Input: part model. Units: mm. Frame: model coordinates. Coordinates: 2 decimals unless noted, no trailing zeros. Order: outer loops, then holes, each group sorted by start corner. A loop starts at its lowest first (then second) coordinate and runs counter-clockwise, first axis right, second up. Notation, with made-up numbers: (34.25, 11.25) - (42.25, 11.25) arc R19 ccw to (42.25, 22.25) - close; hole circle Ø3 at (-21.5, 8.25). An arc over 180 degrees is marked (long way). One line per question, with ' | ' between items.
from build123d import *

# Parameters (mm, degrees)
SKETCH1_W           = 112
SKETCH1_H           = 70
SKETCH1_R           = 1.5
BOSS_EXTRUDE1_DEPTH = 6
SKETCH2_R           = 1.5
CUT_EXTRUDE1_DEPTH  = 85.504437753
SKETCH3_W           = 14
SKETCH3_H           = 6
CUT_EXTRUDE2_DEPTH  = 85.504437753
SKETCH4_R           = 1.5
CUT_EXTRUDE3_DEPTH  = 85.504437753
SKETCH5_R           = 12
CUT_EXTRUDE4_DEPTH  = 85.504437753
SKETCH6_R           = 1.5
CUT_EXTRUDE5_DEPTH  = 10
SKETCH7_W           = 40
SKETCH7_H           = 27.8
BOSS_EXTRUDE2_DEPTH = 6
SKETCH8_W           = 12
SKETCH8_H           = 6
CUT_EXTRUDE6_DEPTH  = 6
SKETCH9_R           = 1.5
CUT_EXTRUDE7_DEPTH  = 6


with BuildPart() as part:
    # Sketch1 → Boss-Extrude1 (new body)
    with BuildSketch(Plane(origin=(0, 0, 0), x_dir=(1, 0, 0), z_dir=(0, 1, 0))):
        with Locations((0, 28)):
            Rectangle(SKETCH1_W, SKETCH1_H)
        with Locations(Location((-6.2, 0, 0), (0, 0, 270))):
            Circle(SKETCH1_R, mode=Mode.SUBTRACT)
        with Locations(Location((-38.2, 0, 0), (0, 0, 270))):
            Circle(SKETCH1_R, mode=Mode.SUBTRACT)
        with Locations(Location((-6.2, 56, 0), (0, 0, 270))):
            Circle(SKETCH1_R, mode=Mode.SUBTRACT)
        with Locations(Location((-38.2, 56, 0), (0, 0, 270))):
            Circle(SKETCH1_R, mode=Mode.SUBTRACT)
        with Locations(Location((6.2, 0, 0), (0, 0, 90))):
            Circle(SKETCH1_R, mode=Mode.SUBTRACT)
        with Locations(Location((38.2, 0, 0), (0, 0, 90))):
            Circle(SKETCH1_R, mode=Mode.SUBTRACT)
        with Locations(Location((6.2, 56, 0), (0, 0, 90))):
            Circle(SKETCH1_R, mode=Mode.SUBTRACT)
        with Locations(Location((38.2, 56, 0), (0, 0, 90))):
            Circle(SKETCH1_R, mode=Mode.SUBTRACT)
    extrude(amount=BOSS_EXTRUDE1_DEPTH)

    # Sketch2 → Cut-Extrude1 (cut, through all)
    with BuildSketch(Plane(origin=(0, 6, 0), x_dir=(1, 0, 0), z_dir=(0, 1, 0))):
        with Locations(Location((-53, 48, 0), (0, 0, 270))):
            Circle(SKETCH2_R)
        with Locations(Location((-53, 8, 0), (0, 0, 270))):
            Circle(SKETCH2_R)
        with Locations(Location((53, 8, 0), (0, 0, 270))):
            Circle(SKETCH2_R)
        with Locations(Location((53, 48, 0), (0, 0, 270))):
            Circle(SKETCH2_R)
    extrude(amount=-CUT_EXTRUDE1_DEPTH, mode=Mode.SUBTRACT)

    # Sketch3 → Cut-Extrude2 (cut, through all)
    with BuildSketch(Plane(origin=(0, 6, 0), x_dir=(1, 0, 0), z_dir=(0, 1, 0))):
        with Locations((20.2, 56)):
            Rectangle(SKETCH3_W, SKETCH3_H)
        with Locations((20.2, 0)):
            Rectangle(SKETCH3_W, SKETCH3_H)
        with Locations((-20.2, 0)):
            Rectangle(SKETCH3_W, SKETCH3_H)
        with Locations((-20.2, 56)):
            Rectangle(SKETCH3_W, SKETCH3_H)
    extrude(amount=-CUT_EXTRUDE2_DEPTH, mode=Mode.SUBTRACT)

    # Sketch4 → Cut-Extrude3 (cut, through all)
    with BuildSketch(Plane(origin=(0, 6, 0), x_dir=(1, 0, 0), z_dir=(0, 1, 0))):
        with Locations(Location((19, 9, 0), (0, 0, 270))):
            Circle(SKETCH4_R)
        with Locations(Location((19, 47, 0), (0, 0, 90))):
            Circle(SKETCH4_R)
        with Locations(Location((-19, 47, 0), (0, 0, 270))):
            Circle(SKETCH4_R)
        with Locations(Location((-19, 9, 0), (0, 0, 90))):
            Circle(SKETCH4_R)
    extrude(amount=-CUT_EXTRUDE3_DEPTH, mode=Mode.SUBTRACT)

    # Sketch5 → Cut-Extrude4 (cut, through all)
    with BuildSketch(Plane(origin=(0, 6, 0), x_dir=(1, 0, 0), z_dir=(0, 1, 0))):
        with Locations(Location((-23, 28, 0), (0, 0, 270))):
            Circle(SKETCH5_R)
        with Locations(Location((23, 28, 0), (0, 0, 270))):
            Circle(SKETCH5_R)
    extrude(amount=-CUT_EXTRUDE4_DEPTH, mode=Mode.SUBTRACT)

    # Sketch6 → Cut-Extrude5 (cut)
    with BuildSketch(Plane(origin=(0, 6, 0), x_dir=(1, 0, 0), z_dir=(0, 1, 0))):
        with Locations(Location((-52, 59, 0), (0, 0, 270))):
            Circle(SKETCH6_R)
        with Locations(Location((52, 59, 0), (0, 0, 270))):
            Circle(SKETCH6_R)
        with Locations(Location((52, -3, 0), (0, 0, 270))):
            Circle(SKETCH6_R)
        with Locations(Location((-52, -3, 0), (0, 0, 270))):
            Circle(SKETCH6_R)
    extrude(amount=-CUT_EXTRUDE5_DEPTH, mode=Mode.SUBTRACT)

    # Sketch7 → Boss-Extrude2 (add)
    with BuildSketch(Plane(origin=(0, 0, 0), x_dir=(1, 0, 0), z_dir=(0, 1, 0))):
        with Locations((-0.079368114, 76.9)):
            Rectangle(SKETCH7_W, SKETCH7_H)
    extrude(amount=BOSS_EXTRUDE2_DEPTH)

    # Sketch8 → Cut-Extrude6 (cut)
    with BuildSketch(Plane(origin=(0, 6, 0), x_dir=(1, 0, 0), z_dir=(0, 1, 0))):
        with Locations((-0.079368114, 81.8)):
            Rectangle(SKETCH8_W, SKETCH8_H)
    extrude(amount=-CUT_EXTRUDE6_DEPTH, mode=Mode.SUBTRACT)

    # Sketch9 → Cut-Extrude7 (cut)
    with BuildSketch(Plane(origin=(0, 6, 0), x_dir=(1, 0, 0), z_dir=(0, 1, 0))):
        with Locations(Location((-17.079368114, 87.8, 0), (0, 0, 270))):
            Circle(SKETCH9_R)
        with Locations(Location((16.920631886, 87.8, 0), (0, 0, 270))):
            Circle(SKETCH9_R)
    extrude(amount=-CUT_EXTRUDE7_DEPTH, mode=Mode.SUBTRACT)


solid = part.part
Item 1: Section A-A on x = 38.2. Return the cut outline in (y, z), and give its area (3 significant figures).
Data:
outline: (0, -63) - (6, -63) - (6, -57.5) - (0, -57.5) - close; (0, -54.5) - (6, -54.5) - (6, -1.5) - (0, -1.5) - close; (0, 1.5) - (6, 1.5) - (6, 7) - (0, 7) - close | area: 384 mm^2
Item 2: Draft query along Z for faces 1 (the face through (19.921, 3, -77)), 2 (the face through (-1, 3, 7)), 3 (the face through (-20, 3, 3)). Return one class per face: released by +Z, released by -Z, zero draft, split by the parting line, or undercut.
Data:
face 1: zero draft | face 2: released by +Z | face 3: undercut
Item 3: Section B-B on z = -28. Return the cut outline in (x, y), and give its area (3 significant figures).
Data:
outline: (-56, 0) - (-35, 0) - (-35, 6) - (-56, 6) - close; (-11, 0) - (11, 0) - (11, 6) - (-11, 6) - close; (35, 0) - (56, 0) - (56, 6) - (35, 6) - close | area: 384 mm^2
Item 4: Section C-C on x = -23. Return the cut outline in (y, z), and give its area (3 significant figures).
Data:
outline: (0, -63) - (6, -63) - (6, -59) - (0, -59) - close; (0, -53) - (6, -53) - (6, -40) - (0, -40) - close; (0, -16) - (6, -16) - (6, -3) - (0, -3) - close; (0, 3) - (6, 3) - (6, 7) - (0, 7) - close | area: 204 mm^2
Item 5: Section D-D on x = -46. Return the cut outline in (y, z), and give its area (3 significant figures).
Data:
outline: (0, -63) - (6, -63) - (6, 7) - (0, 7) - close | area: 420 mm^2
Item 6: Ray query, line 1 (X direction, y = 2.15, z = -87.8); line 2 (X direction, y = 1.5, z = -48); line 3 (X direction, y = 4.9, z = -27.5). Return the intervals inside material, ascending.
Data:
line 1: -20.08 to -18.58, -15.58 to 15.42, 18.42 to 19.92 | line 2: -56 to -54.5, -51.5 to -20.12, -17.88 to 17.88, 20.12 to 51.5, 54.5 to 56 | line 3: -56 to -34.99, -11.01 to 11.01, 34.99 to 56
